Could you check a few things on this model? Use its own coordinates, in mm. Give positions to 0.01 mm unless a question says otherwise; leave off trailing zeros. Loops run counter-clockwise (first coordinate to the right, second up) from the corner with the lowest first, then second, coordinate; pieces in that order, holes last. Notation, with made-up numbers: M 36.25,42.25 L 93.25,42.25 A13 cw 93.25,64.25 Z; hole C -13,10.25 d4. An arc over 180 degrees is marked long. Use CSV: the item, a comma, the result in double quotes.
```python
from build123d import *

# Parameters (mm, degrees)
SKETCH_1_R          = 1.85
SKETCH_1_R_2        = 1.8
SKETCH_1_W          = 40.374860346
SKETCH_1_H          = 10.321291022
SKETCH_1_W_2        = 22
SKETCH_1_H_2        = 5
SKETCH_1_W_3        = 11.667697598
SKETCH_1_H_3        = 6.517356375
EXTRUDE_1_DEPTH     = 3
SKETCH_2_W          = 75.93825213
SKETCH_2_H          = 5.545458332
EXTRUDE_2_DEPTH     = 8
SKETCH_3_R          = 1.8
CUT_EXTRUDE_1_DEPTH = 15


with BuildPart() as part:
    # 草图1 → 凸台-拉伸1 (new body)
    with BuildSketch(Plane(origin=(0, 0, 0), x_dir=(1, 0, 0), z_dir=(0, 1, 0))):
        with BuildLine():
            Line((49.5, -40), (-49.5, -40))
            ThreePointArc((-49.5, -40), (-50.914213562, -39.414213562), (-51.5, -38))
            Line((-51.5, -38), (-51.5, 38))
            ThreePointArc((-51.5, 38), (-50.914213562, 39.414213562), (-49.5, 40))
            Line((-49.5, 40), (49.5, 40))
            ThreePointArc((49.5, 40), (50.914213562, 39.414213562), (51.5, 38))
            Line((51.5, 38), (51.5, -38))
            ThreePointArc((51.5, -38), (50.914213562, -39.414213562), (49.5, -40))
        make_face()
        with Locations(Location((-48.296806281, 36.796806281, 0), (0, 0, 270))):
            Circle(SKETCH_1_R, mode=Mode.SUBTRACT)
        with Locations(Location((48.296806281, 36.796806281, 0), (0, 0, 270))):
            Circle(SKETCH_1_R, mode=Mode.SUBTRACT)
        with Locations(Location((48.296806281, -36.796806281, 0), (0, 0, 270))):
            Circle(SKETCH_1_R, mode=Mode.SUBTRACT)
        with Locations(Location((-48.296806281, -36.796806281, 0), (0, 0, 270))):
            Circle(SKETCH_1_R, mode=Mode.SUBTRACT)
        with Locations(Location((-42.391806281, 12.03, 0), (0, 0, 270))):
            Circle(SKETCH_1_R_2, mode=Mode.SUBTRACT)
        with Locations(Location((-33.901806281, 12.03, 0), (0, 0, 270))):
            Circle(SKETCH_1_R_2, mode=Mode.SUBTRACT)
        with Locations(Location((-33.901806281, -12.03, 0), (0, 0, 270))):
            Circle(SKETCH_1_R_2, mode=Mode.SUBTRACT)
        with Locations(Location((-42.391806281, -12.03, 0), (0, 0, 270))):
            Circle(SKETCH_1_R_2, mode=Mode.SUBTRACT)
        with Locations(Location((33.901806281, -12.03, 0), (0, 0, 270))):
            Circle(SKETCH_1_R_2, mode=Mode.SUBTRACT)
        with Locations(Location((42.391806281, -12.03, 0), (0, 0, 270))):
            Circle(SKETCH_1_R_2, mode=Mode.SUBTRACT)
        with Locations(Location((33.901806281, 12.03, 0), (0, 0, 270))):
            Circle(SKETCH_1_R_2, mode=Mode.SUBTRACT)
        with Locations(Location((42.391806281, 12.03, 0), (0, 0, 270))):
            Circle(SKETCH_1_R_2, mode=Mode.SUBTRACT)
        with Locations((0, 31.409786363)):
            Rectangle(SKETCH_1_W, SKETCH_1_H, mode=Mode.SUBTRACT)
        with Locations((0, -31.19586348)):
            Rectangle(SKETCH_1_W_2, SKETCH_1_H_2, mode=Mode.SUBTRACT)
        with Locations((30.135277266, -31.195863481)):
            Rectangle(SKETCH_1_W_3, SKETCH_1_H_3, mode=Mode.SUBTRACT)
        with Locations((-30.135277266, -31.195863481)):
            Rectangle(SKETCH_1_W_3, SKETCH_1_H_3, mode=Mode.SUBTRACT)
    extrude(amount=EXTRUDE_1_DEPTH)

    # 草图2 → 凸台-拉伸2 (add)
    with BuildSketch(Plane(origin=(0, 3, 0), x_dir=(1, 0, 0), z_dir=(0, 1, 0))):
        with Locations((0, -37.227270834)):
            Rectangle(SKETCH_2_W, SKETCH_2_H)
    extrude(amount=-EXTRUDE_2_DEPTH)

    # 草图3 → 切除-拉伸1 (cut)
    with BuildSketch(Plane(origin=(0, -5, 0), x_dir=(-1, 0, 0), z_dir=(0, -1, 0))):
        with Locations(Location((30.875113943, -37.227270834, 0), (0, 0, 90))):
            Circle(SKETCH_3_R)
        with BuildLine():
            ThreePointArc((10, -37.227270834), (8.2, -35.427270834), (6.4, -37.227270834))
            Line((6.4, -37.227270834), (10, -37.227270834))
        make_face()
        with BuildLine():
            Line((10, -37.227270834), (6.4, -37.227270834))
            ThreePointArc((6.4, -37.227270834), (8.2, -39.027270834), (10, -37.227270834))
        make_face()
        with BuildLine():
            ThreePointArc((-10, -37.227270834), (-8.2, -39.027270834), (-6.4, -37.227270834))
            Line((-6.4, -37.227270834), (-10, -37.227270834))
        make_face()
        with BuildLine():
            Line((-10, -37.227270834), (-6.4, -37.227270834))
            ThreePointArc((-6.4, -37.227270834), (-8.2, -35.427270834), (-10, -37.227270834))
        make_face()
        with Locations(Location((-30.875113943, -37.227270834, 0), (0, 0, 90))):
            Circle(SKETCH_3_R)
    extrude(amount=-CUT_EXTRUDE_1_DEPTH, mode=Mode.SUBTRACT)


solid = part.part
```
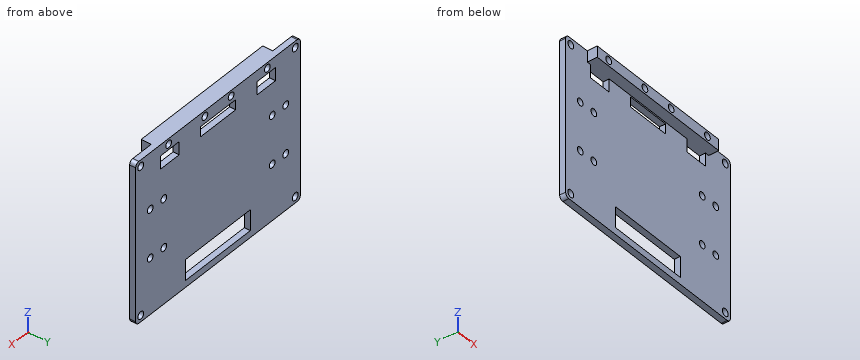
1. I want a section at C-C, the plane x = 18.5. List the corners of the cut face in (y, z) for me.
Outcome:
outline,"M -5,34.45 L 0,34.45 L 0,-26.25 L 3,-26.25 L 3,40 L -5,40 Z; M 0,-40 L 3,-40 L 3,-36.57 L 0,-36.57 Z"
2. I want a section at D-D, the plane y = -3. List the corners of the cut face in (x, z) for me.
Outcome:
outline,"M -37.97,34.45 L 37.97,34.45 L 37.97,40 L -37.97,40 Z; hole C -30.88,37.23 d3.6; hole C -8.2,37.23 d3.6; hole C 8.2,37.23 d3.6; hole C 30.88,37.23 d3.6"
3. I want a section at B-B, the plane z = 12.03. List the corners of the cut face in (x, y) for me, then the cut area to 3 significant figures.
Outcome:
outline,"M -51.5,0 L -44.19,0 L -44.19,3 L -51.5,3 Z; M -40.59,0 L -35.7,0 L -35.7,3 L -40.59,3 Z; M -32.1,0 L 32.1,0 L 32.1,3 L -32.1,3 Z; M 35.7,0 L 40.59,0 L 40.59,3 L 35.7,3 Z; M 44.19,0 L 51.5,0 L 51.5,3 L 44.19,3 Z"
area,"266 mm2"
4. Please list where these lines run through material, in increasing order: line 1 (Z direction, x = 3, y = 1.25); line 2 (Z direction, x = 8.2, y = 0.75); line 3 (Z direction, x = -26, y = 2).
Outcome:
line 1,"-40 to -36.57, -26.25 to 28.7, 33.7 to 40"
line 2,"-40 to -36.57, -26.25 to 28.7, 33.7 to 35.43, 39.03 to 40"
line 3,"-40 to 27.94, 34.45 to 40"
5. I'm going to push flat-ended pins straight in: pin 1 Ø6 at (x, z) = (-33.9, -12.03) entering from -Y; pin 2 Ø3 at (x, y) = (17.5, -3) entering from -Z. Where does each tip first touch, or does it pass through?
Outcome:
pin 1,"y = 0"
pin 2,"z = 34.45"
6. I want a section at A-A, the plane x = -1. List the corners of the cut face in (y, z) for me.
Outcome:
outline,"M -5,34.45 L 0,34.45 L 0,33.7 L 3,33.7 L 3,40 L -5,40 Z; M 0,-40 L 3,-40 L 3,-36.57 L 0,-36.57 Z; M 0,-26.25 L 3,-26.25 L 3,28.7 L 0,28.7 Z"
